from build123d import *

# Parameters (mm, degrees)
ESQUISSE1_W          = 54.61
ESQUISSE1_H          = 37
BOSS_EXTRU_1_DEPTH   = 1.87
ESQUISSE2_R          = 7.93
BOSS_EXTRU_2_DEPTH   = 10.58
ESQUISSE3_W          = 39.43
ESQUISSE3_H          = 1.87
BOSS_EXTRU_3_DEPTH   = 21.15
D_GAGEMENT_M31_D     = 3.6
D_GAGEMENT_M31_DEPTH = 1.99
D_GAGEMENT_M31_TIP   = 1.081549114


with BuildPart() as part:
    # Esquisse1 → Boss.-Extru.1 (new body)
    with BuildSketch(Plane(origin=(0, 0, 0), x_dir=(0, 0, -1), z_dir=(1, 0, 0))):
        with Locations((27.305, 18.5)):
            Rectangle(ESQUISSE1_W, ESQUISSE1_H)
    extrude(amount=BOSS_EXTRU_1_DEPTH)

    # Esquisse2 → Boss.-Extru.2 (add)
    with BuildSketch(Plane(origin=(1.87, 0, 0), x_dir=(0, 0, -1), z_dir=(1, 0, 0))):
        with Locations((13.02, 22.93)):
            Circle(ESQUISSE2_R)
        with Locations((41.59, 22.93)):
            Circle(ESQUISSE2_R)
    extrude(amount=BOSS_EXTRU_2_DEPTH)

    # Esquisse3 → Boss.-Extru.3 (add)
    with BuildSketch(Plane.ZY):
        with Locations((-27.305, 0.935)):
            Rectangle(ESQUISSE3_W, ESQUISSE3_H)
    extrude(amount=BOSS_EXTRU_3_DEPTH)

    # Dégagement M31
    with Locations(Plane(origin=(-18.15, 1.87, -38.5), x_dir=(0, 0, 1), z_dir=(0, 1, 0))):
        with Locations((0, 0), (22.39, 0)):
            Hole(D_GAGEMENT_M31_D / 2, depth=D_GAGEMENT_M31_DEPTH)
            with Locations((0, 0, -(D_GAGEMENT_M31_DEPTH + D_GAGEMENT_M31_TIP / 2))):  # 118° drill point
                Cone(0, D_GAGEMENT_M31_D / 2, D_GAGEMENT_M31_TIP, mode=Mode.SUBTRACT)


solid = part.part
Verification items for the finished model (mm, model axes). A direction names the side the tool comes from. Coordinates: 2 decimals unless noted, no trailing zeros. Order: outer loops, then holes, each group sorted by start corner. A loop starts at its lowest first (then second) coordinate and runs counter-clockwise, first axis right, second up. Notation, with made-up numbers: M 63.25,44 L 67.25,44 A23 ccw 67.25,74 Z; hole C 9.25,29.25 d6. An arc over 180 degrees is marked long. Return JSON: item names as keys, results as strings.
1) Release check for a two-part mould opening along Z. For faces 4 (the cylindrical face through (7.086, 30.793, -11.988)), 5 (the flat face through (-10, 1, -7.59)), 6 (the flat face through (-10, 1.87, -28)) record: +Z half, -Z half, draft (parallel to the pull), parting line (faces both ways), or undercut.
Answer list:
{"face 4": "undercut", "face 5": "+Z half", "face 6": "draft"}
2) Cross-section at B-B, the plane z = -41.59. Record the boundary of the cut face in (x, y).
Answer list:
{"outline": "M -21.15,0 L 1.87,0 L 1.87,15 L 12.45,15 L 12.45,30.86 L 1.87,30.86 L 1.87,37 L 0,37 L 0,1.87 L -21.15,1.87 Z"}
3) Cross-section at C-C, the plane y = 21.5. Record the boundary of the cut face in (x, z).
Answer list:
{"outline": "M 0,-54.61 L 1.87,-54.61 L 1.87,-49.39 L 12.45,-49.39 L 12.45,-33.79 L 1.87,-33.79 L 1.87,-20.82 L 12.45,-20.82 L 12.45,-5.22 L 1.87,-5.22 L 1.87,0 L 0,0 Z"}
4) Gauge pin test, flat ends, axial feed: pin 1 (4 mm diameter, centred on x = 4, y = 24.5, fed in from +Z); pin 2 (2 mm diameter, centred on x = -18.15, z = -38.5, fed in from +Y); pin 3 (6.5 mm diameter, centred on x = -8, z = -27.5, fed in from +Y); pin 4 (8 mm diameter, centred on x = 8, y = 31, fed in from +Z). Record the tip position at first contact, or that the pin passes through.
Answer list:
{"pin 1": "z = -5.09", "pin 2": "through", "pin 3": "y = 1.87", "pin 4": "z = -6.21"}
5) Cross-section at D-D, the plane z = -16.11. Record the boundary of the cut face in (x, y).
Answer list:
{"outline": "M -21.15,0 L -19.95,0 L -19.95,1.87 L -21.15,1.87 Z; M -16.35,0 L 1.87,0 L 1.87,15.63 L 12.45,15.63 L 12.45,30.23 L 1.87,30.23 L 1.87,37 L 0,37 L 0,1.87 L -16.35,1.87 Z"}
6) Thickness scan on L1, parallel to Z at x = -18, y = 1; L2, parallel to X at y = 1.5, z = -16.11; L3, parallel to Y at x = -3, z = -40. Record the ranges inside material, lowest first. Write a range as [from, to].
Answer list:
{"L1": "[-47.02, -40.29], [-36.71, -17.9], [-14.32, -7.59]", "L2": "[-21.15, -19.95], [-16.35, 1.87]", "L3": "[0, 1.87]"}
7) Cross-section at A-A, the plane x = -18.15. Record the boundary of the cut face in (y, z), and give its area (3 significant figures).
Answer list:
{"outline": "M 0,-47.02 L 1.87,-47.02 L 1.87,-40.3 L 0,-40.3 Z; M 0,-36.7 L 1.87,-36.7 L 1.87,-17.91 L 0,-17.91 Z; M 0,-14.31 L 1.87,-14.31 L 1.87,-7.59 L 0,-7.59 Z", "area": "60.3 mm2"}
8) Access from +Z, -Z, +X, -X, +Y, -Y to the whole of each face (thin tool, end or side, straight path). Record for faces 1 (the flat face through (-10, 1, -47.02)), 2 (the flat face through (1, 18, 0)), 3 (the flat face through (1.87, 19, -27)).
Answer list:
{"face 1": "-Z, -X, +Y, -Y", "face 2": "+Z, +X, -X, +Y, -Y", "face 3": "+X"}
